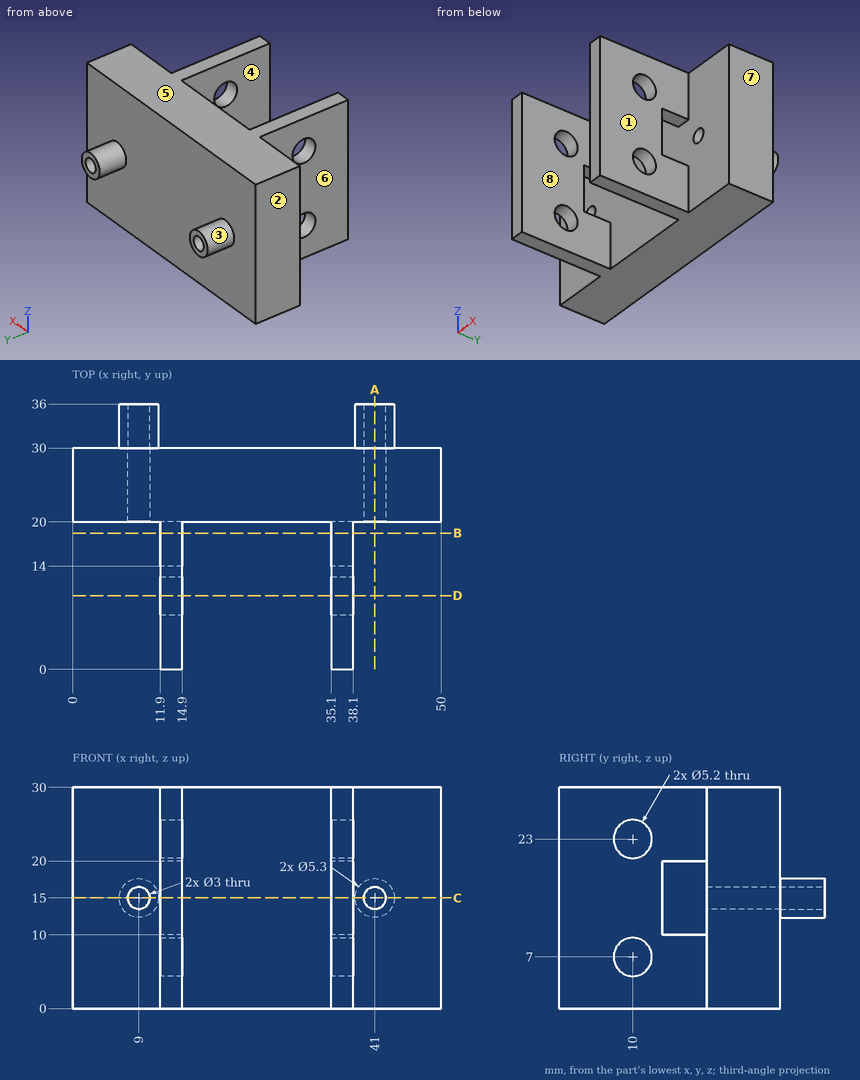
Drawing for the job (mm, zero at the part's lowest x, y, z). A direction names the side the tool comes from. Give positions to 0.01 mm unless a question says otherwise; leave off trailing zeros. Write each loop counter-clockwise with the first axis right and the second up, starting at its lowest first coordinate (ties: lowest second). Pieces come first, ordered by that corner, then holes. Notation, with made-up numbers: (46.5, 28) -> (50.5, 28) arc R13 cw to (50.5, 41) -> close; hole circle Ø2 at (52, 71). An arc over 180 degrees is marked (long way). Put each result on its own line as item: value. Start each with the question number.
Item 1: Pull direction X, two halves, no side cores. Call the marked faces 5, 6, 7 and 8: pulls with the +X half, pulls with the -X half, needs draft (parallel to the pull), parting line crosses it, or undercut.
Item 2: Cut at B-B (y = 18.5). List the corners of the cut face in (x, z).
Item 3: Cut at A-A (x = 41). List the corners of the cut face in (y, z).
Item 4: Cut at D-D (y = 10). List the corners of the cut face in (x, z).
Item 5: Wall check: L1, parallel to X at y = 34.45, z = 15; L2, parallel to X at y = 25.5, z = 15; L3, parallel to X at y = 3, z = 13. Give the ranges that are in metal, low to high. Write a range as [from, to].
Item 6: Cut at C-C (z = 15). List the corners of the cut face in (x, y), then the cut area to 3 significant figures.
Item 7: Pin check, flat tips, straight feed: pin 1 Ø3.5 at (x, z) = (9, 15) entering from -Y; pin 2 Ø6 at (x, z) = (6, 23) entering from +Y; pin 3 Ø5 at (y, z) = (15, 7) entering from +X. Stop position of each tip, or through.
Item 8: Which spindle directions (+Z, -Z, +X, -X, +Y, -Y) get a long thin tool onto all of the face, cutting with end or side? Do the marked faces 1, 2, 3 and 4. Say none if no direction does.
Answer list:
1. face 5: needs draft
1. face 6: pulls with the -X half
1. face 7: pulls with the +X half
1. face 8: undercut
2. outline: (11.9, 0) -> (14.9, 0) -> (14.9, 10) -> (11.9, 10) -> close; (11.9, 20) -> (14.9, 20) -> (14.9, 30) -> (11.9, 30) -> close; (35.1, 0) -> (38.1, 0) -> (38.1, 10) -> (35.1, 10) -> close; (35.1, 20) -> (38.1, 20) -> (38.1, 30) -> (35.1, 30) -> close
3. outline: (20, 0) -> (30, 0) -> (30, 12.35) -> (36, 12.35) -> (36, 13.5) -> (20, 13.5) -> close; (20, 16.5) -> (36, 16.5) -> (36, 17.65) -> (30, 17.65) -> (30, 30) -> (20, 30) -> close
4. outline: (11.9, 0) -> (14.9, 0) -> (14.9, 4.4) -> (11.9, 4.4) -> close; (11.9, 9.6) -> (14.9, 9.6) -> (14.9, 20.4) -> (11.9, 20.4) -> close; (11.9, 25.6) -> (14.9, 25.6) -> (14.9, 30) -> (11.9, 30) -> close; (35.1, 0) -> (38.1, 0) -> (38.1, 4.4) -> (35.1, 4.4) -> close; (35.1, 9.6) -> (38.1, 9.6) -> (38.1, 20.4) -> (35.1, 20.4) -> close; (35.1, 25.6) -> (38.1, 25.6) -> (38.1, 30) -> (35.1, 30) -> close
5. L1: x = [6.35, 7.5], [10.5, 11.65], [38.35, 39.5], [42.5, 43.65]
5. L2: x = [0, 7.5], [10.5, 39.5], [42.5, 50]
5. L3: x = [11.9, 14.9], [35.1, 38.1]
6. outline: (0, 20) -> (7.5, 20) -> (7.5, 36) -> (6.35, 36) -> (6.35, 30) -> (0, 30) -> close; (10.5, 20) -> (39.5, 20) -> (39.5, 36) -> (38.35, 36) -> (38.35, 30) -> (11.65, 30) -> (11.65, 36) -> (10.5, 36) -> close; (11.9, 0) -> (14.9, 0) -> (14.9, 14) -> (11.9, 14) -> close; (35.1, 0) -> (38.1, 0) -> (38.1, 14) -> (35.1, 14) -> close; (42.5, 20) -> (50, 20) -> (50, 30) -> (43.65, 30) -> (43.65, 36) -> (42.5, 36) -> close
6. area: 552 mm2
7. pin 1: stops at y = 20
7. pin 2: stops at y = 30
7. pin 3: stops at x = 38.1
8. face 1: +Z, -Z, +X, -Y
8. face 2: +Z, -Z, -X, +Y, -Y
8. face 3: +Y
8. face 4: +Z, -Z, -Y
